Design review of the part built by this model. Coordinates are the model's own, in mm. A direction names the side the tool comes from. Coordinates: 2 decimals unless noted, no trailing zeros. Write each loop counter-clockwise with the first axis right and the second up, starting at its lowest first coordinate (ties: lowest second). Pieces come first, ordered by that corner, then holes. Notation, with made-up numbers: (17, 85) -> (38, 85) arc R9 cw to (38, 97) -> close; hole circle Ø7 at (31.25, -30). An arc over 180 degrees is marked (long way). Answer in a Markdown table with one row per item. Add a question column.
Item 1: Take a section at A-A, the plane x = -37.5. Write out the cut boundary in (y, z), and give its area (3 significant figures).
Item 2: Draft analysis for pull direction X (two halves, no side actions). For faces 3 (the face through (-50, 0, 1)), 4 (the face through (-1, 17, 2)), 5 (the face through (-36.579, 14.655, 1.014)), 6 (the face through (38.421, 14.655, 1.014)), state which applies: released by +X, released by -X, zero draft, split by the parting line, or undercut.
Item 3: Take a section at C-C, the plane z = 1.65. Write out the cut boundary in (x, y), and give its area (3 significant figures).
Item 4: Take a section at D-D, the plane x = -17. Write out the cut boundary in (y, z).
Item 5: For faces 1 (the face through (0, 13, 1)), 2 (the face through (-1, 25, 1)), list the 3-axis set-ups (+Z, -Z, +X, -X, +Y, -Y) from which the entire face can be reached by the end or side of a thin tool; tool diameter is ignored.
Item 6: Take a section at B-B, the plane y = -15.5. Write out the cut boundary in (x, z), and give its area (3 significant figures).
Item 7: To check wall thickness, follow line 1 (Y direction, x = 37.5, z = 0.9); line 2 (X direction, y = -15.5, z = 0.5); line 3 (X direction, y = -0.5, z = 0.9). State the ranges of each line that lie inside material, in increasing order.
Item 8: Clearance check with flat-ended pins moving along their axes: P1, Ø3, axis at x = -37.5, y = -15.5, coming from the -Z side; P2, Ø2, axis at x = 37.5, y = 15.5, coming from the +Z side. State where each tip first meets the part, or that it passes through.
from build123d import *

# Parameters (mm, degrees)
F0_W     = 100
F0_H     = 50
F0_W_2   = 72.5
F0_H_2   = 26.5
F1_DEPTH = 2
F2_D     = 2.5


with BuildPart() as f1:
    # F0 (on Top) → F1 (new body)
    with BuildSketch(Plane.XY):
        Rectangle(F0_W, F0_H)
        with Locations((0.75, -0.25)):
            Rectangle(F0_W_2, F0_H_2, mode=Mode.SUBTRACT)
    extrude(amount=F1_DEPTH)

    # F2 (through all)
    with Locations(Plane(origin=(0, 0, 0), x_dir=(1, 0, 0), z_dir=(0, 0, -1))):
        with Locations((-37.5, -15.5), (-37.5, 15.5), (37.5, 15.5), (37.5, -15.5)):
            Hole(F2_D / 2)


solid = f1.part
Answers:
| question | item | result |
|---|---|---|
| 1 | outline | (-25, 0) -> (-16.75, 0) -> (-16.75, 2) -> (-25, 2) -> close; (-14.25, 0) -> (14.25, 0) -> (14.25, 2) -> (-14.25, 2) -> close; (16.75, 0) -> (25, 0) -> (25, 2) -> (16.75, 2) -> close |
| 1 | area | 90.0 mm^2 |
| 2 | face 3 | released by -X |
| 2 | face 4 | zero draft |
| 2 | face 5 | undercut |
| 2 | face 6 | undercut |
| 3 | outline | (-50, -25) -> (50, -25) -> (50, 25) -> (-50, 25) -> close; hole circle Ø2.5 at (-37.5, -15.5); hole circle Ø2.5 at (-37.5, 15.5); hole (-35.5, -13.5) -> (37, -13.5) -> (37, 13) -> (-35.5, 13) -> close; hole circle Ø2.5 at (37.5, -15.5); hole circle Ø2.5 at (37.5, 15.5) |
| 3 | area | 3,060 mm^2 |
| 4 | outline | (-25, 0) -> (-13.5, 0) -> (-13.5, 2) -> (-25, 2) -> close; (13, 0) -> (25, 0) -> (25, 2) -> (13, 2) -> close |
| 5 | face 1 | +Z, -Z |
| 5 | face 2 | +Z, -Z, +X, -X, +Y |
| 6 | outline | (-50, 0) -> (-38.75, 0) -> (-38.75, 2) -> (-50, 2) -> close; (-36.25, 0) -> (36.25, 0) -> (36.25, 2) -> (-36.25, 2) -> close; (38.75, 0) -> (50, 0) -> (50, 2) -> (38.75, 2) -> close |
| 6 | area | 190 mm^2 |
| 7 | line 1 | y = -25 to -16.75, -14.25 to 14.25, 16.75 to 25 |
| 7 | line 2 | x = -50 to -38.75, -36.25 to 36.25, 38.75 to 50 |
| 7 | line 3 | x = -50 to -35.5, 37 to 50 |
| 8 | P1 | stops at z = 0 |
| 8 | P2 | passes through |
